Could you check a few things on this model? Use its own coordinates, in mm. Face numbers are marked on the shaded views. A direction names the side the tool comes from. Give positions to 0.01 mm unless a question says otherwise; leave off trailing zeros. Order: outer loops, then holes, each group sorted by start corner. A loop starts at its lowest first (then second) coordinate and runs counter-clockwise, first axis right, second up. Notation, with made-up numbers: M 53.5,56.5 L 72.5,56.5 A23 ccw 72.5,85.5 Z; hole C 45,37 d5. An arc over 180 degrees is marked long. Answer in a Markdown table with one row per item. Add a question column.
```python
from build123d import *

# Parameters (mm, degrees)
BOSS_EXTRUDE1_DEPTH     = 18.57
SKETCH2_R               = 3.35
CUT_EXTRUDE1_DEPTH      = 18.57
CUT_EXTRUDE2_REACH      = 23.011
CUT_EXTRUDE2_END_RADIUS = 3.35
SKETCH3_R               = 1.875
FILLET1_R               = 0.18


with BuildPart() as part:
    # Sketch1 → Boss-Extrude1 (new body)
    with BuildSketch(Plane(origin=(0, 0, 0), x_dir=(1, 0, 0), z_dir=(0, 1, 0))):
        with BuildLine():
            Line((2.45, 3.098386677), (2.45, 5.05))
            Line((2.45, 5.05), (-2.45, 5.05))
            Line((-2.45, 5.05), (-2.45, 3.098386677))
            ThreePointArc((-2.45, 3.098386677), (0, -3.95), (2.45, 3.098386677))
        make_face()
    extrude(amount=BOSS_EXTRUDE1_DEPTH)

    # Sketch2 → Cut-Extrude1 (cut)
    with BuildSketch(Plane.XZ):
        with Locations(Location((0, 0, 0), (0, 0, 270))):
            Circle(SKETCH2_R)
    extrude(amount=-CUT_EXTRUDE1_DEPTH, mode=Mode.SUBTRACT)

    # Cut-Extrude2: up to this cylinder (the profile starts outside it)
    cut_extrude2_end = Plane(origin=(0, 9.55, 0), z_dir=(0, -1, 0)) * Cylinder(CUT_EXTRUDE2_END_RADIUS, 66.672, mode=Mode.PRIVATE)
    # Sketch3 → Cut-Extrude2 (cut, up to the surface)
    with BuildSketch(Plane(origin=(0, 0, -5.05), x_dir=(-1, 0, 0), z_dir=(0, 0, -1)), mode=Mode.PRIVATE) as cut_extrude2_sk1:
        with Locations((0, 16.025)):
            Circle(SKETCH3_R)
    cut_extrude2_tool1 = extrude(cut_extrude2_sk1.sketch, amount=-CUT_EXTRUDE2_REACH, mode=Mode.PRIVATE) - cut_extrude2_end
    add(cut_extrude2_tool1.solids().sort_by_distance((0, 16.025, -5.05))[0], mode=Mode.SUBTRACT)
    # Sketch3 → Cut-Extrude2 (cut, up to the surface)
    with BuildSketch(Plane(origin=(0, 0, -5.05), x_dir=(-1, 0, 0), z_dir=(0, 0, -1)), mode=Mode.PRIVATE) as cut_extrude2_sk2:
        with Locations((0, 3.075)):
            Circle(SKETCH3_R)
    cut_extrude2_tool2 = extrude(cut_extrude2_sk2.sketch, amount=-CUT_EXTRUDE2_REACH, mode=Mode.PRIVATE) - cut_extrude2_end
    add(cut_extrude2_tool2.solids().sort_by_distance((0, 3.075, -5.05))[0], mode=Mode.SUBTRACT)

    # Fillet1
    fillet1_edges = [part.edges().sort_by_distance(p)[0] for p in [
        (-2.45, 9.285, -5.05),
        (2.45, 9.285, -5.05),
    ]]
    fillet(fillet1_edges, radius=FILLET1_R)


solid = part.part
```
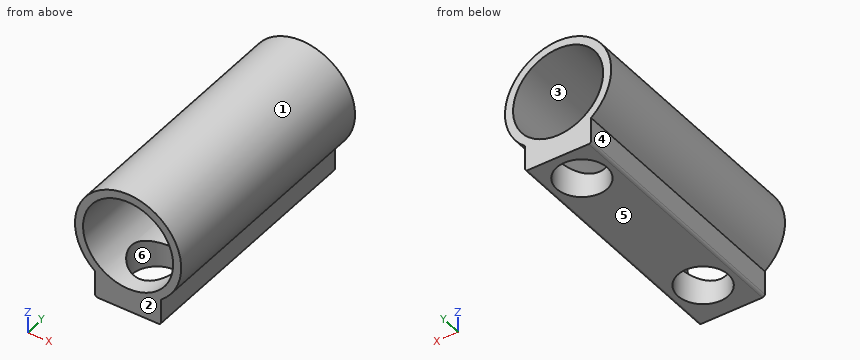
1. Suppose I cut it at A-A on z = 0. List the corners of the cut face in (x, y) for me.
2. For the marked faces 4, 5 and 6, which set-ups out of +Z, -Z, +X, -X, +Y, -Y let a thin tool reach every point of the face, with its end or its side?
3. If I drill on line 1 along Y through (x, z) = (0, -4.15); line 2 along X through (y, z) = (5.75, 0); line 3 along Z through (x, y) = (3, 5.25), over which ranges is the centre line in solid material (lowest first)? Write a range as [from, to].
4. Thinking about a two-plate mould opening in Z: for the marked faces 1, 2 and 3, which applies, pulls with the +Z half, pulls with the -Z half, needs draft (parallel to the pull), parting line crosses it, or undercut?
5. Suppose I cut it at B-B on y = 12. List the corners of the cut face in (x, z) for me.
6. Will these pins go through, and if not, where does the flat tip stop? P1, Ø1.4, axis at y = 13, z = -4, coming from the -X side; P2, Ø5, axis at y = 10, z = -3, coming from the +X side; P3, Ø0.9, axis at y = 7.5, z = -3.5, coming from the +X side; P4, Ø2, axis at x = -1, z = 0, coming from the -Y side.
7. Suppose I cut it at D-D on x = 2.75. List the corners of the cut face in (y, z) for me, plus the area to 3 significant figures.
8. Suppose I cut it at C-C on x = 0. List the corners of the cut face in (y, z) for me.
Findings below:
| question | item | result |
|---|---|---|
| 1 | outline | M -3.95,0 L -3.35,0 L -3.35,18.57 L -3.95,18.57 Z; M 3.35,0 L 3.95,0 L 3.95,18.57 L 3.35,18.57 Z |
| 2 | face 4 | -Z, -X, +Y, -Y |
| 2 | face 5 | -Z, +X, -X, +Y, -Y |
| 2 | face 6 | -Z |
| 3 | line 1 | [0, 1.2], [4.95, 14.15], [17.9, 18.57] |
| 3 | line 2 | [-3.95, -3.35], [3.35, 3.95] |
| 3 | line 3 | [-2.57, -1.49], [1.49, 2.57] |
| 4 | face 1 | parting line crosses it |
| 4 | face 2 | needs draft |
| 4 | face 3 | undercut |
| 5 | outline | M -2.45,-4.87 A0.18 ccw -2.27,-5.05 L 2.27,-5.05 A0.18 ccw 2.45,-4.87 L 2.45,-3.1 A3.95 ccw long -2.45,-3.1 Z; hole C 0,0 d6.7 |
| 6 | P1 | x = -2.45 |
| 6 | P2 | x = 3.92 |
| 6 | P3 | x = 2.51 |
| 6 | P4 | through |
| 7 | outline | M 0,-2.84 L 18.57,-2.84 L 18.57,-1.91 L 0,-1.91 Z; M 0,1.91 L 18.57,1.91 L 18.57,2.84 L 0,2.84 Z |
| 7 | area | 34.3 mm2 |
| 8 | outline | M 0,-5.05 L 1.2,-5.05 L 1.2,-3.35 L 0,-3.35 Z; M 0,3.35 L 18.57,3.35 L 18.57,3.95 L 0,3.95 Z; M 4.95,-5.05 L 14.15,-5.05 L 14.15,-3.35 L 4.95,-3.35 Z; M 17.9,-5.05 L 18.57,-5.05 L 18.57,-3.35 L 17.9,-3.35 Z |
